Read the model definition and answer for the solid it produces. Units are mm, in the model's axes. A direction names the side the tool comes from. Coordinates: 2 decimals unless noted, no trailing zeros. Loops run counter-clockwise (first coordinate to the right, second up) from the corner with the lowest first, then second, coordinate; pieces in that order, holes last. Notation, with made-up numbers: (-26, 44.5) -> (-7, 44.5) arc R29 cw to (-7, 73.5) -> close; hole circle Ø10 at (35, 76.25). An arc over 180 degrees is marked (long way). Answer as CSV lines item,"result".
Autodesk Inventor part; units mm, degrees
ref_plane "Work Plane1" through (0, 0, 0) normal (0.6427876, -0.7660444, 0) x (0, 0, -1)
ref_plane "Work Plane2" through (0, 14.3, -22) normal (0.6427876, 0.7660444, 0) x (0, 0, 1)
ref_plane "YZ Plane" through (0, 0, 0) normal (1, 0, 0) x (0, 1, 0)
sketch "Sketch1" plane through (0, 0, 0) normal (0, 1, 0) x (-1, 0, 0)
  circle A0 centre (0, 0) radius 5.075
  circle A1 centre (0, 0) radius 20
  line L0 (1.5, -3.825) -> (-1.5, -3.825)
  line L1 (-1.5, -3.825) -> (-1.5, -6.325)
  line L2 (-1.5, -6.325) -> (1.5, -6.325)
  line L3 (1.5, -6.325) -> (1.5, -3.825)
  line L4 (1.5, -3.825) -> (-1.5, -6.325) construction
  line L5 (-1.5, -3.825) -> (1.5, -6.325) construction
  circle A2 centre (0, 0) radius 2.5
  circle A3 centre (0, 0) radius 8.754
  point P0 (0, -5.075)
  point P1 (-1.5, -4.8483)
  point P2 (1.5, -4.8483)
  dimension "d0" = 10.15
  dimension "d1" = 40
  dimension "d2" = 1.25
  dimension "d3" = 3
  dimension "d17" = 5
extrude "Extrusion1" add sketch "Sketch1" along normal blind 14.3 contours A1 | A3
sketch "Sketch2" plane through (0, 0, 0) normal (1, 0, 0) x (0, 1, 0)
  line L0 (0, 0) -> (14.3, 0)
  line L1 (14.3, 0) -> (14.3, -22)
  line L2 (14.3, -22) -> (0, -22) construction
  line L3 (0, -22) -> (0, 0)
  line L4 (0, -22) -> (14.3, -22) construction
  line L5 (14.3, -22) -> (14.3, -20.0661)
  line L6 (0, -20) -> (14.3, -20)
  circle A0 centre (7.15, -22) radius 2.5
  line L7 (9.65, -22) -> (4.65, -22)
  line L8 (4.65, -22) -> (4.65, -26)
  line L9 (4.65, -26) -> (9.65, -26)
  line L10 (9.65, -26) -> (9.65, -22)
  line L11 (14.3, -20) -> (0, -20)
  line L12 (0, -20) -> (0, -26)
  line L13 (0, -26) -> (14.3, -26)
  line L14 (14.3, -26) -> (14.3, -20)
  point P0 (5.65, -20)
  point P1 (14.3, -22)
  point P2 (14.3, -20)
  point P3 (8.65, -20)
  point P4 (14.3, -20)
  point P5 (8.65, -20)
  dimension "d22" = 5
  dimension "d7" = 22
  dimension "d10" = 14.3
  dimension "d23" = 4
  dimension "d31" = 6
  dimension "d41" = 14.3
  dimension "d42" = 5
revolve "Revolution1" add sketch "Sketch2" angle 360 about axis through (0, 0, 0) along (0, 1, 0) contours L0 L1 L6 A0 L3 | L6 A0 L8 L13 L12 L3 | L1 L14 L13 L10 A0 L6 | A0 L6
extrude "Extrusion3" add sketch "Sketch1" against normal blind 2 contours A0 L3 L0 L1 | L1 L0 L3 A0 | A0 L3 L2 L1 | A3
revolve "Revolution4" cut sketch "Sketch2" angle 360 about axis through (0, 0, 0) along (0, 1, 0) contours A0 L6
sketch "Sketch3" plane through (0, 0, 0) normal (0, -1, 0) x (1, 0, 0)
  line L0 (0, 0) -> (0, -22)
  dimension "d25" = 22
ref_plane "Work Plane1" through (0, 0, 0) normal (0.6427876, -0.7660444, 0) x (0, 0, -1)
sketch "Sketch4" plane through (0, 0, 0) normal (0.6427876, -0.7660444, 0) x (0, 0, -1)
  ellipse E0 centre (0, 2.7318) end of major axis (22, 2.7318) minor radius 16.853
  line L0 (0, 0) -> (22, 0)
  circle A0 centre (22, 0) radius 2
  dimension "d27" = 22
  dimension "d28" = 4
extrude "Extrusion4" cut sketch "Sketch4" against normal blind 9 contours A0 L0 E0 | E0 A0 | E0 L0 A0 picked at (22.5049, 0.1658)
extrude "Extrusion5" cut sketch "Sketch4" along normal blind 7 contours A0 L0 E0 | E0 A0 | E0 L0 A0 picked at (22.5049, 0.1658)
ref_plane "Work Plane2" through (0, 14.3, -22) normal (0.6427876, 0.7660444, 0) x (0, 0, 1)
sketch "Sketch5" plane through (0, 14.3, -22) normal (0.6427876, 0.7660444, 0) x (0, 0, 1)
  ellipse E0 centre (22, -0.5142) end of major axis (27.075, -0.5142) minor radius 3.8877 (17.1517, -1.6633) -> (17.1517, 0.6348) ccw
  line L0 (22, -0.5142) -> (0, -0.5142)
  circle A0 centre (0, -0.5142) radius 2
  point P0 (22, 9.1919)
  dimension "d35" = 22
  dimension "d36" = 4
extrude "Extrusion6" cut sketch "Sketch5" against normal blind 9
extrude "Extrusion7" cut sketch "Sketch5" along normal blind 8
extrude "Extrusion8" cut sketch "Sketch1" along normal through all contours A0 L3 L0 L1 | L1 L0 L3 A0 | A0 L3 L2 L1 | A2
sketch "Sketch6" plane through (0, 14.3, 0) normal (0, 1, 0) x (1, 0, 0)
  circle A0 centre (0, 0) radius 15
  circle A1 centre (0, 0) radius 35.6972
  dimension "d45" = 30
extrude "Extrusion9" cut sketch "Sketch6" against normal blind 2.5
sketch "Sketch7" plane through (0, 0, 0) normal (0, -1, 0) x (1, 0, 0)
  circle A0 centre (0, 0) radius 2.5
  circle A1 centre (0, 0) radius 20
  line L0 (24, -7.5) -> (-24, -7.5)
  line L1 (-24, -7.5) -> (-24, 7.5)
  line L2 (-24, 7.5) -> (24, 7.5)
  line L3 (24, 7.5) -> (24, -7.5)
  line L4 (24, -7.5) -> (-24, 7.5) construction
  line L5 (-24, -7.5) -> (24, 7.5) construction
  circle A2 centre (0, 0) radius 11
  circle A3 centre (20, 0) radius 1.75
  circle A4 centre (-20, 0) radius 1.75
  dimension "d48" = 40
  dimension "d49" = 48
  dimension "d50" = 15
  dimension "d51" = 22
  dimension "d52" = 3.5
  dimension "d53" = 3.5
extrude "Extrusion10" cut sketch "Sketch7" against normal blind 4 contours A1 A3 | A1 A3 | A4 A1 | A1 A4
properties part number "spool"
Q1. For faces 5 (the face through (1.898, -0.986, -8.546)), 6 (the face through (1.5, 7, -6)), 7 (the face through (-17.5, 9.65, 13.6)), 8 (the face through (-2, -2, -2)), determine the directions among +Z, -Z, +X, -X, +Y, -Y from which every point of the face is accessible in a straight line to the end or side of a thin tool.
Results:
face 5,"-Y"
face 6,"+Y"
face 7,"none"
face 8,"+Z, -Z, +X, -X, -Y"
Q2. A cutting plane is placed at A-A, the plane y = 7.25. Write down the section's boundary in (x, z) (3 decimals).
Results:
outline,"circle Ø39.004 at (0, 0); hole (-1.5, -6.325) -> (1.5, -6.325) -> (1.5, -4.848) arc R5.075 ccw (long way) to (-1.5, -4.848) -> close"
Q3. For a pull along Y with two mould halves and no side action, classify faces 1 (the face through (-13.6, 4.65, 17.5)), 2 (the face through (-20, 4, 0)), 3 (the face through (-3.183, 10.372, -20.092)), 4 (the face through (0, 7, -6.325)) as pulls with the +Y half, pulls with the -Y half, needs draft (parallel to the pull), parting line crosses it, or undercut.
Results:
face 1,"undercut"
face 2,"pulls with the -Y half"
face 3,"undercut"
face 4,"needs draft"
Q4. Find the intervals of material crossed by probe 1 along X at (y, z) = (3.1, 0) (3 decimals); probe 2 along Y at (x, z) = (-11.5, -19); probe 3 along Z at (x, y) = (0, -1.4), in increasing order. Write a range as [from, to].
Results:
probe 1,"x = [-26, -21.75], [-18.25, -5.075], [5.075, 18.25], [21.75, 26]"
probe 2,"y = [0, 4.65], [9.65, 11.8]"
probe 3,"z = [-8.75, -2.5], [2.5, 8.75]"
Q5. Given pin 1 Ø1 at (x, z) = (-20.5, 0) entering from -Y; pin 2 Ø8 at (x, z) = (0, 0) entering from +Y; pin 3 Ø10 at (x, z) = (-7.5, -5.5) entering from -Y; pin 4 Ø10 at (x, z) = (2, -18) entering from -Y, each flat-ended and moving along its own axis, determine where each tip first touches the part or whether it passes through.
Results:
pin 1,"stops at y = 4"
pin 2,"stops at y = 0"
pin 3,"stops at y = -2"
pin 4,"stops at y = 0"
